```python
from build123d import *

# Parameters (mm, degrees)
F0_R     = 32.75
F0_R_2   = 26.1
F1_DEPTH = 1.65
F2_W     = 5
F2_H     = 5
F3_DEPTH = 1.62
F4_COUNT = 24


with BuildPart() as f1:
    # F0 (on Top) → F1 (new body)
    with BuildSketch(Plane.XY):
        Circle(F0_R)
        Circle(F0_R_2, mode=Mode.SUBTRACT)
    extrude(amount=F1_DEPTH)

    # F2 (on face) → F3 (join)
    with BuildSketch(Plane.XY.offset(1.65)):
        with Locations((0, -29)):
            Rectangle(F2_W, F2_H)
    extrude(amount=F3_DEPTH)

    # F4: F1 ×24 about axis
    f4_axis = Axis((0, 0, 1.65), (0, 0, 1))


with BuildPart() as f1_1:
    add(f1.part)
    for i in range(1, F4_COUNT):
        add(f1.part.rotate(f4_axis, i * 360 / F4_COUNT))


solid = f1_1.part
```
Can you work these out from the model? Positions are in its coordinate system, mm. A direction names the side the tool comes from. Coordinates: 2 decimals unless noted, no trailing zeros. Loops run counter-clockwise (first coordinate to the right, second up) from the corner with the lowest first, then second, coordinate; pieces in that order, holes last. Notation, with made-up numbers: M 4,-17 L 60,-17 A32 cw 60,14 Z; hole C 42,-27.75 d10. An arc over 180 degrees is marked long. Put each result on its own line as item: value. Start each with the question number.
(1) Imagine slicing it at A-A on y = 0. List the corners of the cut face in (x, z) for me, and give its area (3 significant figures).
(2) Imagine slicing it at C-C on z = 2.75. Give the number of separate pieces and of enclosed holes in the cut face, and give its area (3 significant figures).
(3) Will these pins go through, and if not, where does the flat tip stop? pin 1 Ø0.8 at (x, z) = (-1, 2) entering from -Y; pin 2 Ø0.5 at (x, z) = (-29.5, 2) entering from -Y; pin 3 Ø1.3 at (x, z) = (29, 2.5) entering from +Y; pin 4 Ø1.5 at (x, y) = (22, 14) entering from +Z.
(4) I need wall thicknesses on probe 1 along X at (y, z) = (0, 0.75); probe 2 along X at (y, z) = (-27, 3.05). Which ranges of each line are inside material? Lowest first, please.
(5) Which directions (+Z, -Z, +X, -X, +Y, -Y) give clear straight access to the entire face, cutting with the end or side of a thin tool? Please do faces 1 (the face through (-30.418, 8.187, 2.449)), 2 (the face through (-30.436, -8.119, 2.449)), 3 (the face through (12.352, 26.395, 2.449)), 4 (the face through (-22.299, 18.763, 2.449)), 5 (the face through (-28.7, -5.1, 2.4)).
(6) Imagine slicing it at D-D on x = -27.5. List the corners of the cut face in (y, z) for me, and give its area (3 significant figures).
(7) We'd pull the mould along Y, two halves only. Please class faces 6 (the face through (-5.1, -28.7, 2.4)), 7 (the face through (31.5, 0, 2)), 8 (the face through (-25.606, -6.825, 2.449)), 9 (the face through (13.22, -22.967, 2.449)): +Y half, -Y half, draft (parallel to the pull), parting line (faces both ways), or undercut.
Worked answers:
1. outline: M -32.75,0 L -26.1,0 L -26.1,1.65 L -26.5,1.65 L -26.5,3.27 L -31.5,3.27 L -31.5,1.65 L -32.75,1.65 Z; M 26.1,0 L 32.75,0 L 32.75,1.65 L 31.5,1.65 L 31.5,3.27 L 26.5,3.27 L 26.5,1.65 L 26.1,1.65 Z
1. area: 38.1 mm2
2. separate pieces: 24
2. enclosed holes: 0
2. area: 600 mm2
3. pin 1: stops at y = -32.74
3. pin 2: stops at y = -10.56
3. pin 3: stops at y = 13.9
3. pin 4: stops at z = 3.27
4. probe 1: x = -32.75 to -26.1, 26.1 to 32.75
4. probe 2: x = -16.23 to -12.7, -9.82 to -4.65, -2.5 to 2.5, 4.65 to 9.82, 12.7 to 16.23
5. face 1: +Z, -X, +Y
5. face 2: +Z, -X, -Y
5. face 3: +Z, +Y
5. face 4: +Z
5. face 5: +Z, -X
6. outline: M -17.79,0 L 17.79,0 L 17.79,1.65 L 15.37,1.65 L 15.37,3.27 L 12.99,3.27 L 12.99,1.65 L 9.96,1.65 L 9.96,3.27 L 4.78,3.27 L 4.78,1.65 L 2.5,1.65 L 2.5,3.27 L -2.5,3.27 L -2.5,1.65 L -4.78,1.65 L -4.78,3.27 L -9.96,3.27 L -9.96,1.65 L -12.99,1.65 L -12.99,3.27 L -15.37,3.27 L -15.37,1.65 L -17.79,1.65 Z
6. area: 91.3 mm2
7. face 6: -Y half
7. face 7: draft
7. face 8: undercut
7. face 9: undercut
